Can you work these out from the model? Positions are in its coordinate system, mm. Face numbers are marked on the shaded views. A direction names the side the tool comes from. Coordinates: 2 decimals unless noted, no trailing zeros. Order: outer loops, then holes, each group sorted by start corner. A loop starts at its lowest first (then second) coordinate and runs counter-clockwise, first axis right, second up. Notation, with made-up numbers: (11, -3) - (53, -3) arc R5 cw to (53, 1) - close; hole circle Ø10 at (19, -8.5). An arc over 180 degrees is marked (long way). Return JSON: item names as keys, results as strings. Group by question number.
1) For pin 1 Ø2 at (y, z) = (-40, 21.5) entering from -X; pin 2 Ø1.5 at (y, z) = (-3, 6) entering from +X; pin 3 Ø12.5 at (x, y) = (2, 7) entering from +Z, each with a flat end and sliding along its axis, tell me the tip position at first contact or that it passes through.
2) Imagine slicing it at C-C (y = -3.5). Write out the boundary of the cut face in (x, z).
3) If we mould it in two halves opening along Y, with no side actions, what happens to the marked faces 1, 2 and 3? For each: pulls with the +Y half, pulls with the -Y half, needs draft (parallel to the pull), parting line crosses it, or undercut.
4) Imagine slicing it at D-D (z = 10). Write out the boundary of the cut face in (x, y).
5) Imagine slicing it at A-A (z = 23.25). Write out the boundary of the cut face in (x, y).
6) Imagine slicing it at B-B (x = -2.5). Write out the boundary of the cut face in (y, z).
7) If I drill on line 1 along X through (y, z) = (22, 9.75); line 2 along Y through (x, z) = (26, 19.75); line 3 along Y through (x, z) = (-35, 16.25), over which ranges is the centre line in solid material (lowest first)?
8) Which directions (+Z, -Z, +X, -X, +Y, -Y) give clear straight access to the entire face, cutting with the end or side of a thin tool? Please do the marked faces 4, 5 and 6.
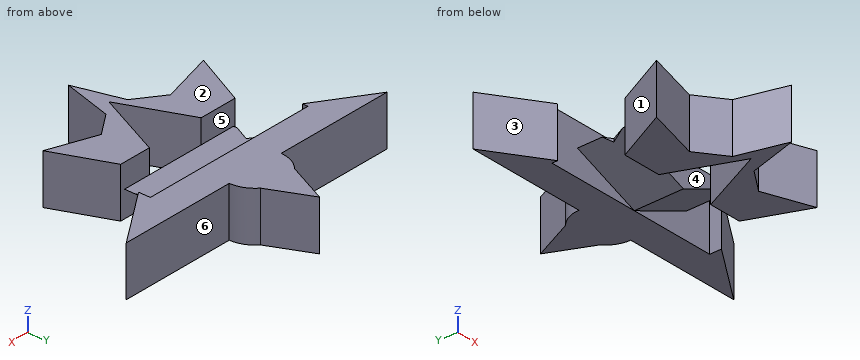
```python
from build123d import *

# Parameters (mm, degrees)
F0_W     = 14.3528226763
F0_H     = 40.9249328077
F0_W_2   = 15.9044768661
F1_DEPTH = 25.4
F3_DEPTH = 36.322
F5_DEPTH = 25.146


with BuildPart() as f1:
    # F0 (on Top) → F1 (new body)
    with BuildSketch(Plane.XY):
        with Locations((-7.1764113382, 20.4624664038)):
            Rectangle(F0_W, F0_H)
        with Locations((7.9522384331, 20.4624664038)):
            Rectangle(F0_W_2, F0_H)
        Polygon((-29.3328283983, 9.9198052494), (-14.3528226763, 0), (-14.3528226763, 40.9249328077), align=None)
        Polygon((-5.9702647759, -30.3703169913), (-14.3528226763, 0), (-47.713432461, -28.1237699091), (-19.6796488017, -20.3861221671), align=None)
        Polygon((-47.713432461, -28.1237699091), (-14.3528226763, 0), (-29.3328283983, 9.9198052494), align=None)
        Polygon((0, -34.7183085978), (-14.3528226763, 0), (-5.9702647759, -30.3703169913), align=None)
        with BuildLine():
            Line((-14.3528226763, 40.9249328077), (0, 40.9249328077))
            Line((0, 40.9249328077), (15.9044768661, 40.9249328077))
            Line((15.9044768661, 40.9249328077), (10.6561835989, 52.3815727712))
            ThreePointArc((10.6561835989, 52.3815727712), (0.7758270949, 56.0535825789), (-9.1045294091, 52.3815727712))
            Line((-9.1045294091, 52.3815727712), (-14.3528226763, 40.9249328077))
        make_face()
        Polygon((28.9926118268, 8.9120575126), (15.9044768661, 0), (44.6101129055, -29.2875114828), align=None)
        Polygon((7.8085155122, -29.3319671142), (15.9044768661, 0), (0, -34.7183085978), align=None)
        Polygon((15.9044768661, 40.9249328077), (15.9044768661, 0), (28.9926118268, 8.9120575126), align=None)
        Polygon((44.6101129055, -29.2875114828), (15.9044768661, 0), (7.8085155122, -29.3319671142), (20.5186381936, -20.5644797534), align=None)
        Polygon((-29.3328283983, 9.9198052494), (-14.3528226763, 40.9249328077), (-76.1540085077, 40.9249328077), align=None)
        with BuildLine():
            ThreePointArc((-9.1045294091, 52.3815727712), (-12.9783085934, 47.2257101699), (-14.3528226763, 40.9249328077))
            Line((-14.3528226763, 40.9249328077), (-9.1045294091, 52.3815727712))
        make_face()
        Polygon((7.8085155122, -29.3319671142), (0, -34.7183085978), (-5.9702647759, -30.3703169913), (0.7758270949, -54.8116570932), align=None)
        Polygon((76.0063156486, 40.9249328077), (15.9044768661, 40.9249328077), (28.9926118268, 8.9120575126), align=None)
        with BuildLine():
            Line((10.6561835989, 52.3815727712), (15.9044768661, 40.9249328077))
            ThreePointArc((15.9044768661, 40.9249328077), (14.5299627832, 47.2257101699), (10.6561835989, 52.3815727712))
        make_face()
        with BuildLine():
            Line((0.7758270949, 73.9496676573), (-9.1045294091, 52.3815727712))
            ThreePointArc((-9.1045294091, 52.3815727712), (0.7758270949, 56.0535825789), (10.6561835989, 52.3815727712))
            Line((10.6561835989, 52.3815727712), (0.7758270949, 73.9496676573))
        make_face()
    extrude(amount=F1_DEPTH)

    # F2 (on Top) → F3 (cut)
    with BuildSketch(Plane.XY):
        Polygon((0, 17.6911037415), (0, 0), (26.803391082, 17.6601352598), align=None)
        Polygon((-27.6542542717, 17.7230553056), (0, 0), (0, 17.6911037415), align=None)
        Polygon((-44.7053313255, 28.6507476121), (-27.6542542717, 17.7230553056), (0, 17.6911037415), align=None)
        Polygon((0, 17.6911037415), (26.803391082, 17.6601352598), (43.3298423886, 28.5490322858), align=None)
        Polygon((-44.7053313255, 28.6507476121), (0, 17.6911037415), (43.3298423886, 28.5490322858), align=None)
    extrude(amount=-F3_DEPTH, mode=Mode.SUBTRACT)

    # F4 (on Front) → F5 (cut)
    with BuildSketch(Plane.XZ):
        with BuildLine():
            Line((43.9610369503, 0), (0, 0))
            Line((0, 0), (-48.0021461844, 0))
            ThreePointArc((-48.0021461844, 0), (-2.020554617, -23.4103047443), (43.9610369503, 0))
        make_face()
        Polygon((30.382517891, 13.2921541349), (0, 0), (43.9610369503, 0), (43.9610369503, 19.2326679826), align=None)
        Polygon((-48.0021461844, 0), (0, 0), (-33.1754245675, 13.2921541349), (-48.0021461844, 19.2326679826), align=None)
        Polygon((-48.0021461844, 19.2326679826), (-33.1754245675, 13.2921541349), (0, 13.2921541349), (0, 36.8990898132), align=None)
        Polygon((0, 13.2921541349), (30.382517891, 13.2921541349), (43.9610369503, 19.2326679826), (0, 36.8990898132), align=None)
        Polygon((-48.0021461844, 56.3966855407), (-48.0021461844, 19.2326679826), (0, 36.8990898132), (43.9610369503, 19.2326679826), (43.9610369503, 56.5599761903), (0, 56.3966855407), align=None)
    extrude(amount=-F5_DEPTH, mode=Mode.SUBTRACT)


solid = f1.part
```
Calculated:
{
 "1": {"pin 1": "x = -3.59", "pin 2": "x = 34.17", "pin 3": "z = 13.29"},
 "2": {"outline": "(-35.82, 0) - (-12.91, 0) - (-12.91, 25.4) - (-35.82, 25.4) - close; (14.3, 0) - (34.07, 0) - (34.07, 25.4) - (14.3, 25.4) - close"},
 "3": {"face 1": "undercut", "face 2": "needs draft", "face 3": "pulls with the -Y half"},
 "4": {"outline": "(-76.15, 40.92) - (-48, 22.28) - (-48, 25.15) - (-24.96, 25.15) - (-24.96, 0) - (-34.13, 0) - (-47.71, -28.12) - (-19.68, -20.39) - (-5.97, -30.37) - (0.78, -54.81) - (7.81, -29.33) - (20.52, -20.56) - (44.61, -29.29) - (32.64, 0) - (22.86, 0) - (22.86, 25.15) - (43.96, 25.15) - (43.96, 19.1) - (76.01, 40.92) - (15.9, 40.92) arc R15.13 ccw to (10.66, 52.38) - (0.78, 73.95) - (-9.1, 52.38) arc R15.13 ccw to (-14.35, 40.92) - close; hole (-14.35, 0) - (0, -34.72) - (15.9, 0) - close"},
 "5": {"outline": "(-76.15, 40.92) - (-48, 22.28) - (-48, 25.15) - (43.96, 25.15) - (43.96, 19.1) - (76.01, 40.92) - (15.9, 40.92) arc R15.13 ccw to (10.66, 52.38) - (0.78, 73.95) - (-9.1, 52.38) arc R15.13 ccw to (-14.35, 40.92) - close; (-47.71, -28.12) - (-19.68, -20.39) - (-5.97, -30.37) - (0.78, -54.81) - (7.81, -29.33) - (20.52, -20.56) - (44.61, -29.29) - (32.64, 0) - (15.9, 0) - (0, -34.72) - (-14.35, 0) - (-34.13, 0) - close"},
 "6": {"outline": "(-42.94, 0) - (-28.67, 0) - (-28.67, 25.4) - (-42.94, 25.4) - close; (0, 1) - (25.15, 1) - (25.15, 0) - (66.8, 0) - (66.8, 25.4) - (25.15, 25.4) - (25.15, 13.29) - (0, 13.29) - close"},
 "7": {"line 1": "-24.33 to 22.29, 43.96 to 48.21", "line 2": "-22.55 to 0, 25.15 to 40.92", "line 3": "-24.61 to -1.81, 25.15 to 40.92"},
 "8": {"face 4": "+Z, -Z", "face 5": "-X", "face 6": "+Z, -Z, +X, +Y"}
}
